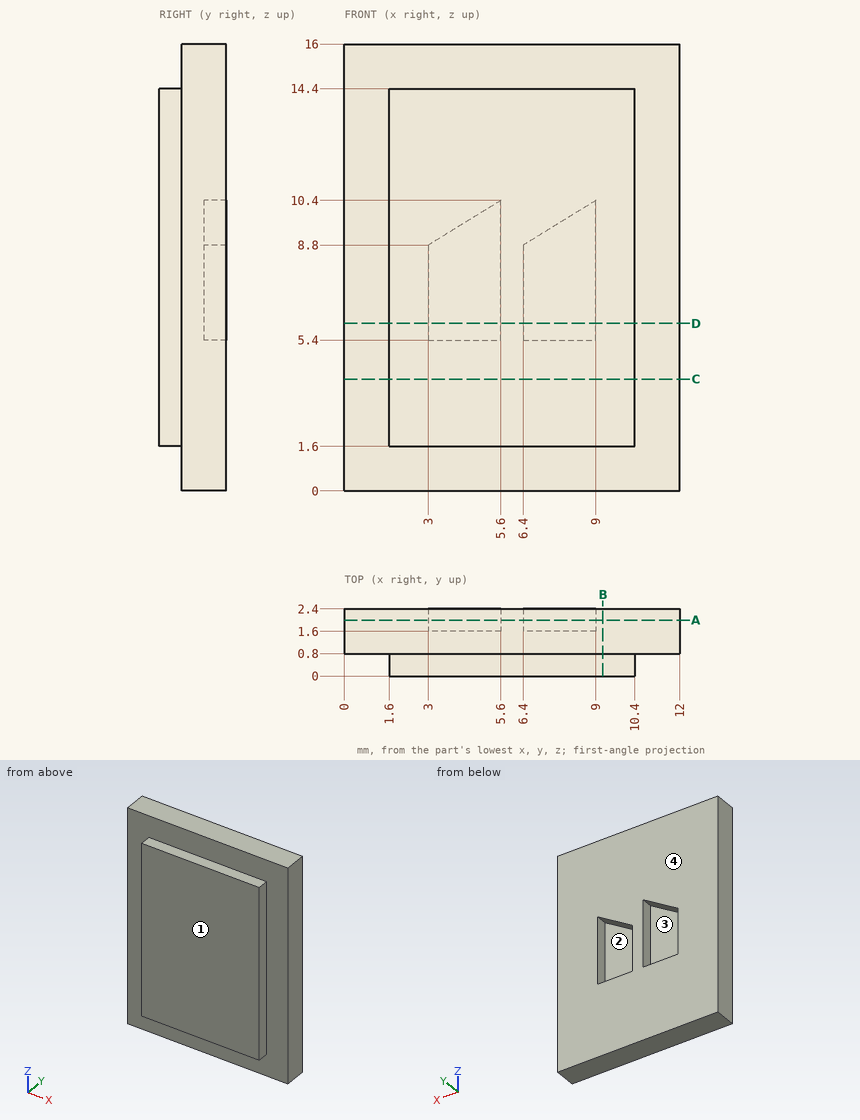
Input: dimensioned drawing with shaded views. Units: mm. Origin: part minimum x, y, z. A direction names the side the tool comes from. Give positions to 0.01 mm unless a question says otherwise; leave off trailing zeros. Write each loop counter-clockwise with the first axis right and the second up, starting at its lowest first coordinate (ties: lowest second). Pieces come first, ordered by that corner, then holes. Notation, with made-up numbers: (65, 89.25) -> (108, 89.25) arc R17 cw to (108, 100.25) -> close; hole circle Ø9 at (77, 55). An arc over 180 degrees is marked (long way). Return JSON: item names as keys, results as strings. Group by question number.
1. Section D-D, the plane z = 6. Output: boundary loops of the cut face in (x, y).
2. Section B-B, the plane x = 9.25. Output: boundary loops of the cut face in (y, z), then the cut area to 3 significant figures.
3. Pin query (flat end, axial travel): pin 1 Ø4 at (x, z) = (2.5, 2) entering from -Y; pin 2 Ø0.8 at (x, z) = (8.5, 7) entering from +Y. Return the tip coordinate at first contact, or that it passes through.
4. Access query for the marked faces 3 and 4. Directions: +Z, -Z, +X, -X, +Y, -Y. A direction counts if a zero-diameter tool reaches every point of the face in a straight line with its end or side. Return the directions, or none.
5. Material intervals for line 1 (Y direction, x = 8.25, z = 15.25); line 2 (X direction, y = 0.6, z = 12.5); line 3 (Z direction, x = 3.5, y = 1.65), sorted ascending. Write a range as from..to.
6. Mould query, pull axis Z, two halves, no side actions, for the marked faces 1 and 2. Classes: +Z half, -Z half, draft (parallel to the pull), parting line (faces both ways), or undercut.
7. Section A-A, the plane y = 2. Output: boundary loops of the cut face in (x, z).
8. Section C-C, the plane z = 4. Output: boundary loops of the cut face in (x, y).
Determined:
{
 "1": {"outline": "(0, 0.8) -> (1.6, 0.8) -> (1.6, 0) -> (10.4, 0) -> (10.4, 0.8) -> (12, 0.8) -> (12, 2.4) -> (9, 2.4) -> (9, 1.6) -> (6.4, 1.6) -> (6.4, 2.4) -> (5.6, 2.4) -> (5.6, 1.6) -> (3, 1.6) -> (3, 2.4) -> (0, 2.4) -> close"},
 "2": {"outline": "(0, 1.6) -> (0.8, 1.6) -> (0.8, 0) -> (2.4, 0) -> (2.4, 16) -> (0.8, 16) -> (0.8, 14.4) -> (0, 14.4) -> close", "area": "35.8 mm2"},
 "3": {"pin 1": "stops at y = 0", "pin 2": "stops at y = 1.6"},
 "4": {"face 3": "+Y", "face 4": "+Z, -Z, +X, -X, +Y"},
 "5": {"line 1": "y = 0.8..2.4", "line 2": "x = 1.6..10.4", "line 3": "z = 0..5.4, 9.11..16"},
 "6": {"face 1": "draft", "face 2": "undercut"},
 "7": {"outline": "(0, 0) -> (12, 0) -> (12, 16) -> (0, 16) -> close; hole (3, 5.4) -> (5.6, 5.4) -> (5.6, 10.4) -> (3, 8.8) -> close; hole (6.4, 5.4) -> (9, 5.4) -> (9, 10.4) -> (6.4, 8.8) -> close"},
 "8": {"outline": "(0, 0.8) -> (1.6, 0.8) -> (1.6, 0) -> (10.4, 0) -> (10.4, 0.8) -> (12, 0.8) -> (12, 2.4) -> (0, 2.4) -> close"}
}
